from build123d import *

# Parameters (mm, degrees)
EXTRUDE1_DEPTH      = 4.365625
SKETCH2_W           = 1.7526
SKETCH2_H           = 4.365625
LPATTERN1_COUNT     = 6
LPATTERN1_PITCH     = 0.79375
LPATTERN1_COL_COUNT = 2
LPATTERN1_COL_PITCH = 0.79375
SKETCH8_R           = 2.192732982
BOSS_EXTRUDE1_DEPTH = 3.714221


with BuildPart() as part:
    # Sketch1 → Extrude1 (new body)
    with BuildSketch(Plane(origin=(0, 0, 0), x_dir=(1, 0, 0), z_dir=(0, 1, 0))):
        Polygon((0, 4.582717762), (-3.96875, 2.291358881), (-3.96875, -2.291358881), (0, -4.582717762), (3.96875, -2.291358881), (3.96875, 2.291358881), align=None)
    extrude(amount=EXTRUDE1_DEPTH)

    # Sketch4 → Cut-Revolve2 (revolve, cut)
    with BuildSketch(Plane(origin=(0, 0, 0), x_dir=(0, 0, -1), z_dir=(1, 0, 0))):
        Polygon((0, 4.365625), (1.7526, 4.365625), (1.410275607, 4.205996514), (1.410275607, 0.159628486), (1.7526, 0), (0, 0), align=None)
    revolve(axis=Axis((0, 4.365625, 0), (0, 1, 0)), mode=Mode.SUBTRACT)


with BuildPart() as body_2:
    # Sketch2 → Revolve1 (revolve)
    with BuildSketch(Plane(origin=(0, 0, 0), x_dir=(0, 0, -1), z_dir=(1, 0, 0))):
        with Locations((0.8763, 2.1828125)):
            Rectangle(SKETCH2_W, SKETCH2_H)
    revolve(axis=Axis((0, -1.7526, 0), (0, 1, 0)))

    # Sketch3 → Cut-Revolve1 (revolve, cut)
    with BuildSketch(Plane(origin=(0, 0, 0), x_dir=(0, 0, -1), z_dir=(1, 0, 0))):
        Polygon((1.774513192, 4.268856346), (1.927905533, 3.591475768), (1.454101991, 3.7385105), (1.410275607, 3.932047808), align=None)
    cut_revolve1 = revolve(axis=Axis((0, 4.365625, 0.193538035), (0, -0.975306119, -0.220857364)), mode=Mode.SUBTRACT)

    # LPattern1: Cut-Revolve1 ×6
    with Locations(*[(0, -i * LPATTERN1_PITCH, 0) for i in range(1, LPATTERN1_COUNT)]):
        add(cut_revolve1, mode=Mode.SUBTRACT)

    # LPattern1 col: Cut-Revolve1 ×2
    with Locations(*[(0, i * LPATTERN1_COL_PITCH, 0) for i in range(1, LPATTERN1_COL_COUNT)]):
        add(cut_revolve1, mode=Mode.SUBTRACT)


with BuildPart() as part_1:
    add(part.part)

    # Combine1: cut body 2
    add(body_2.part, mode=Mode.SUBTRACT)

    # Sketch5 → Cut-Revolve3 (revolve, cut)
    with BuildSketch(Plane(origin=(0, 0, 0), x_dir=(0, 0, -1), z_dir=(1, 0, 0))):
        with BuildLine():
            Line((0, 0), (3.96875, 0))
            Line((3.96875, 0), (4.582717762, 0.286297869))
            Line((4.582717762, 0.286297869), (4.582717762, 3.351722964))
            Line((4.582717762, 3.351722964), (3.96875, 3.638020833))
            ThreePointArc((3.96875, 3.638020833), (3.755639674, 4.152514674), (3.241145833, 4.365625))
            Line((3.241145833, 4.365625), (3.241145833, 5.635625))
            Line((3.241145833, 5.635625), (5.852717762, 5.635625))
            Line((5.852717762, 5.635625), (5.852717762, -1.27))
            Line((5.852717762, -1.27), (0, -1.27))
            Line((0, -1.27), (0, 0))
        make_face()
    revolve(axis=Axis((0, 0, 0), (0, 1, 0)), mode=Mode.SUBTRACT)

    # Sketch6 → Cut-Revolve4 (revolve, cut)
    with BuildSketch(Plane(origin=(0, 0, 0), x_dir=(0, 0, -1), z_dir=(1, 0, 0))):
        with BuildLine():
            Line((0, 3.638020833), (3.81635, 3.638020833))
            ThreePointArc((3.81635, 3.638020833), (3.6478766, 4.0447516), (3.241145833, 4.213225))
            Line((3.241145833, 4.213225), (2.32571072, 4.213225))
            Line((2.32571072, 4.213225), (2.32571072, 5.635625))
            Line((2.32571072, 5.635625), (0, 5.635625))
            Line((0, 5.635625), (0, 3.638020833))
        make_face()
    revolve(axis=Axis((0, 5.635625, 0), (0, 1, 0)), mode=Mode.SUBTRACT)



with BuildPart() as body_2_2:
    # Sketch7 → Revolve2 (revolve)
    with BuildSketch(Plane(origin=(0, 0, 0), x_dir=(0, 0, -1), z_dir=(1, 0, 0))):
        with BuildLine():
            Line((1.410275607, 3.714220833), (3.734297654, 3.714220833))
            ThreePointArc((3.734297654, 3.714220833), (3.565938876, 4.016854092), (3.241145833, 4.137025))
            Line((3.241145833, 4.137025), (1.410275607, 4.137025))
            Line((1.410275607, 4.137025), (1.410275607, 3.714220833))
        make_face()
    revolve(axis=Axis((0, 3.714220833, 0), (0, 1, 0)))


with BuildPart() as part_2:
    add(part_1.part)

    add(body_2_2.part)  # Boss-Extrude1 merges body 2 2
    # Sketch8 → Boss-Extrude1 (add)
    with BuildSketch(Plane.XZ):
        Circle(SKETCH8_R)
    extrude(amount=-BOSS_EXTRUDE1_DEPTH)

    # Sketch10 → #6-32 Tapped Hole1 (revolve, cut)
    with BuildSketch(Plane(origin=(0, 3.714220833, 0), x_dir=(0, 0, 1), z_dir=(1, 0, 0))):
        Polygon((0, 0), (0, 3.714220833), (1.98755, 3.714220833), (1.35255, 3.079220833), (1.35255, 0), align=None)
    revolve(axis=Axis((0, 10.064220833, 0), (0, -1, 0)), mode=Mode.SUBTRACT)


solid = part_2.part
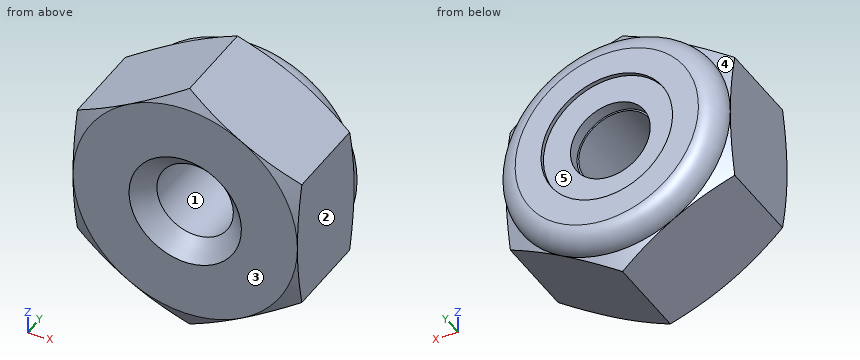
Source: CAD feature listing. Evaluate the final solid. Frame: model axes, mm. Face numbers are marked on the shaded views. A direction names the side the tool comes from. Round coordinates to 2 decimals unless told otherwise and drop trailing zeros. Write each loop counter-clockwise with the first axis right and the second up, starting at its lowest first coordinate (ties: lowest second). Pieces come first, ordered by that corner, then holes. Notation, with made-up numbers: M 17,85.5 L 51,85.5 A21 cw 51,120.5 Z; hole C 35.5,-29.75 d11. An arc over 180 degrees is marked long. One line per item, written item: value. Start each with the question number.
Item 1: Mould query, pull axis X, two halves, no side actions, for the marked faces 1, 2 and 3. Classes: pulls with the +X half, pulls with the -X half, needs draft (parallel to the pull), parting line crosses it, or undercut.
Item 2: Set-up query: the marked faces 4 and 5. Return all of +Z, -Z, +X, -X, +Y, -Y with unobstructed straight access to the full face (end or side cutting, diameter ignored); none if empty.
Item 3: Section query B-B (z = 2.75). State how many separate pieces and enclosed holes the cut face has, plus the area to 3 significant figures.
Item 4: Pin query (flat end, axial travel): pin 1 (3.5 mm diameter, centred on x = 0, z = 0, fed in from -Y); pin 2 (3.5 mm diameter, centred on x = 0, z = 0, fed in from +Y); pin 3 (2.5 mm diameter, centred on x = 0, z = 0, fed in from +Y); pin 4 (1 mm diameter, centred on x = 1, y = 2, fed in from -Z). Return the tip coordinate at first contact, or that it passes through.
Item 5: Section query A-A (y = 2.7). Return the cut outline in (x, z).
Item 6: Ray query, L1, parallel to X at y = 1.95, z = 0; L2, parallel to X at y = 1, z = -0.5; L3, parallel to Z at x = 0, y = 4.25. Return the intervals inside material, ascending. Write a range as from..to.
Result set:
1. face 1: undercut
1. face 2: pulls with the +X half
1. face 3: needs draft
2. face 4: +Z, -X, +Y
2. face 5: none
3. separate pieces: 2
3. enclosed holes: 1
3. area: 26.0 mm²
4. pin 1: stops at y = 0.24
4. pin 2: stops at y = 4.14
4. pin 3: passes through
4. pin 4: stops at z = -4.29
5. outline: M -3.97,-2.29 L 0,-4.58 L 3.97,-2.29 L 3.97,2.29 L 0,4.58 L -3.97,2.29 Z; hole C 0,0 d2.71
6. L1: x = -3.97..-1.35, 1.35..3.97
6. L2: x = -3.97..-1.26, 1.26..3.97
6. L3: z = -3.63..-2.33, 2.33..3.63
